Here's how the part is built. I have some questions about the finished solid (model axes, mm). A direction names the side the tool comes from. Coordinates: 2 decimals unless noted, no trailing zeros. Write each loop counter-clockwise with the first axis right and the second up, starting at its lowest first coordinate (ties: lowest second). Pieces come first, ordered by that corner, then holes.
from build123d import *

# Parameters (mm, degrees)
SKETCH2_W                = 100
SKETCH2_H                = 3
SKETCH2_H_2              = 11
BOSS_EXTRUDE2_DEPTH      = 2
SKETCH3_W                = 100
SKETCH3_H                = 3
BOSS_EXTRUDE3_DEPTH      = 20
FILLET2_R                = 1
BOSS_EXTRUDE5_DEPTH      = 30
BOSS_EXTRUDE5_DEPTH_BACK = 1
SKETCH5_W                = 9.5
SKETCH5_H                = 10
FILLET3_R                = 2
FILLET4_R                = 2
SKETCH6_R                = 2
CUT_EXTRUDE1_DEPTH       = 39
SKETCH7_R                = 2
CUT_EXTRUDE2_DEPTH       = 39


# Some blends are built 0.0001 mm under size
with BuildPart() as part:
    # Sketch2 → Boss-Extrude2 (new body)
    with BuildSketch(Plane(origin=(0, 0, 0), x_dir=(1, 0, 0), z_dir=(0, 1, 0))):
        with Locations((-50, 1.5)):
            Rectangle(SKETCH2_W, SKETCH2_H)
        with Locations((-50, -5.5)):
            Rectangle(SKETCH2_W, SKETCH2_H_2)
        with Locations((-50, -12.5)):
            Rectangle(SKETCH2_W, SKETCH2_H)
    extrude(amount=BOSS_EXTRUDE2_DEPTH)

    # Sketch3 → Boss-Extrude3 (add)
    with BuildSketch(Plane(origin=(0, 2, 0), x_dir=(1, 0, 0), z_dir=(0, 1, 0))):
        with Locations((-50, -12.5)):
            Rectangle(SKETCH3_W, SKETCH3_H)
        with Locations((-50, 1.5)):
            Rectangle(SKETCH3_W, SKETCH3_H)
    extrude(amount=BOSS_EXTRUDE3_DEPTH)

    # Fillet2
    fillet2_edges = [part.edges().sort_by_distance(p)[0] for p in [
        (-100, 11, -3),
        (0, 11, -3),
        (0, 11, 14),
        (-100, 11, 14),
        (-100, 2, 5.5),
        (0, 2, 5.5),
        (0, 12, 11),
        (-100, 12, 11),
        (-100, 22, 12.5),
        (0, 22, 12.5),
        (-50, 2, 11),
        (-50, 2, 0),
        (-100, 12, 0),
        (0, 12, 0),
        (-100, 22, -1.5),
        (0, 22, -1.5),
        (-50, 0, -3),
        (0, 0, 5.5),
        (-50, 0, 14),
        (-100, 0, 5.5),
    ]]
    fillet(fillet2_edges, radius=FILLET2_R - 0.0001)  # a hair under: the kernel refuses the full size

    # Sketch5 → Boss-Extrude5 (add, two sides: drawn at the far end of the back side and taken through both)
    with BuildSketch(Plane(origin=(0, 0, -3), x_dir=(-1, 0, 0), z_dir=(0, 0, -1)).offset(-BOSS_EXTRUDE5_DEPTH_BACK)):
        with Locations((50, 5)):
            Rectangle(SKETCH5_W, SKETCH5_H)
    extrude(amount=BOSS_EXTRUDE5_DEPTH + BOSS_EXTRUDE5_DEPTH_BACK)

    # Fillet3
    fillet3_edges = [part.edges().sort_by_distance(p)[0] for p in [
        (-45.25, 5, -33),
        (-50, 0, -33),
        (-54.75, 5, -33),
        (-50, 10, -33),
    ]]
    fillet(fillet3_edges, radius=FILLET3_R)

    # Fillet4
    # the kernel refuses this fillet: 2 mm, written as the material it adds along each edge
    with BuildSketch(Plane(origin=(-54.75, 0.9999, -2.0001), x_dir=(0, 0.0062831439655585564, -0.9999802608561371), z_dir=(0, -0.9999802608561371, -0.0062831439655585564))) as fillet4_piece_1_section:
        with BuildLine():
            CenterArc((-0.9999 - FILLET4_R, -FILLET4_R), FILLET4_R, 0, 90)
            Line((-0.9999, -FILLET4_R), (-0.9999, 0))
            Line((-0.9999, 0), (-0.9999 - FILLET4_R, 0))
        make_face()
    fillet4_piece_1 = revolve(axis=Axis((-54.75, 0.9999, -2.0001), (1, 0, 0)), revolution_arc=359.64, mode=Mode.PRIVATE)
    fillet4_piece_1 = split(fillet4_piece_1, bisect_by=Plane(origin=(-55.461006322, 0, -2.760267515), z_dir=(0, 1, 0)), keep=Keep.TOP, mode=Mode.PRIVATE)
    fillet4_piece_1 = split(fillet4_piece_1, bisect_by=Plane(origin=(-55.461006322, 0.239732481, 0), z_dir=(0, 0, -1)), keep=Keep.TOP, mode=Mode.PRIVATE)
    add(fillet4_piece_1)
    with BuildSketch(Plane(origin=(-45.25, 0.9999, -2.0001), x_dir=(0, 0.0062831439655585564, -0.9999802608561371), z_dir=(0, -0.9999802608561371, -0.0062831439655585564))) as fillet4_piece_2_section:
        with BuildLine():
            CenterArc((-0.9999 - FILLET4_R, FILLET4_R), FILLET4_R, 270, 90)
            Line((-0.9999, FILLET4_R), (-0.9999, 0))
            Line((-0.9999, 0), (-0.9999 - FILLET4_R, 0))
        make_face()
    fillet4_piece_2 = revolve(axis=Axis((-45.25, 0.9999, -2.0001), (1, 0, 0)), revolution_arc=359.64, mode=Mode.PRIVATE)
    fillet4_piece_2 = split(fillet4_piece_2, bisect_by=Plane(origin=(-44.538993678, 0, -2.760267519), z_dir=(0, 1, 0)), keep=Keep.TOP, mode=Mode.PRIVATE)
    fillet4_piece_2 = split(fillet4_piece_2, bisect_by=Plane(origin=(-44.538993678, 0.239732485, 0), z_dir=(0, 0, -1)), keep=Keep.TOP, mode=Mode.PRIVATE)
    add(fillet4_piece_2)
    with BuildSketch(Plane(origin=(-45.25, 10, -3), x_dir=(0, 0, -1), z_dir=(0, -1, 0)), Plane(origin=(-54.75, 0.9999, -3), x_dir=(0, 0, -1), z_dir=(0, 1, 0))) as fillet4_piece_3:
        with BuildLine():
            CenterArc((FILLET4_R, FILLET4_R), FILLET4_R, 180, 90)
            Line((0, FILLET4_R), (0, 0))
            Line((0, 0), (FILLET4_R, 0))
        make_face()
    extrude(amount=9.0001)

    # Sketch6 → Cut-Extrude1 (cut)
    with BuildSketch(Plane(origin=(0, 0, -3), x_dir=(-1, 0, 0), z_dir=(0, 0, -1))):
        with Locations((17.333333335, 18)):
            Circle(SKETCH6_R)
        with Locations((50.000000335, 18)):
            Circle(SKETCH6_R)
        with Locations((82.666667335, 18)):
            Circle(SKETCH6_R)
    extrude(amount=-CUT_EXTRUDE1_DEPTH, mode=Mode.SUBTRACT)

    # Sketch7 → Cut-Extrude2 (cut)
    with BuildSketch(Plane(origin=(0, 10, 0), x_dir=(1, 0, 0), z_dir=(0, 1, 0))):
        with Locations(Location((-50, 11, 0), (0, 0, 270))):
            Circle(SKETCH7_R)
    extrude(amount=-CUT_EXTRUDE2_DEPTH, mode=Mode.SUBTRACT)


solid = part.part
1. Thinking about a two-plate mould opening in Z: for faces 6 (the face through (-51, 11, 14)), 7 (the face through (-48.526, 19.352, 12.479)), 8 (the face through (-50, 5, -33)), 9 (the face through (-51, 12, 11)), which applies, pulls with the +Z half, pulls with the -Z half, needs draft (parallel to the pull), parting line crosses it, or undercut?
2. I want a section at D-D (x = -65). List the corners of the cut face in (y, z) for me.
3. For pin 1 Ø3 at (x, y) = (-50, 18) entering from -Z; pin 2 Ø3 at (y, z) = (3.5, -17.5) entering from -X; pin 3 Ø5 at (x, y) = (-42, 9.5) entering from -Z; pin 4 Ø4.5 at (x, y) = (-17.33, 18) entering from -Z, each with a flat end and sliding along its axis, tell me the tip position at first contact or that it passes through.
4. I want a section at B-B (z = -11). List the corners of the cut face in (x, y) for me.
5. I want a section at C-C (x = -50). List the corners of the cut face in (y, z) for me.
6. On a 3-axis mill with a long thin cutter (end or side, diameter ignored), from which of +Z, -Z, +X, -X, +Y, -Y can I reach the whole of each face in a straight line? I mean faces 1 (the face through (-54.75, 5, -18)), 2 (the face through (-45.25, 5, -18)), 3 (the face through (-51, 12, 0)), 4 (the face through (-19.24, 18.6, -1.52)), 5 (the face through (-50, 10, -17)). Say none if no direction works.
7. I want a section at A-A (y = 7). List the corners of the cut face in (x, z) for me.
8. If I drill on line 1 (Z direction, x = -43, y = 16.5); line 2 (Y direction, x = -50, z = 11.9); line 3 (Y direction, x = -51.5, z = -21.5), over which ranges is the centre line in solid material (lowest first)?
Response values:
1. face 6: pulls with the +Z half
1. face 7: needs draft
1. face 8: pulls with the -Z half
1. face 9: undercut
2. outline: (0, -2) arc R1 ccw to (1, -3) - (22, -3) - (22, 0) - (3, 0) arc R1 cw to (2, 1) - (2, 10) arc R1 cw to (3, 11) - (22, 11) - (22, 14) - (1, 14) arc R1 ccw to (0, 13) - close
3. pin 1: passes through
3. pin 2: stops at x = -54.75
3. pin 3: stops at z = -3.44
3. pin 4: stops at z = -3
4. outline: (-54.75, 0) - (-52, 0) - (-52, 10) - (-54.75, 10) - close; (-48, 0) - (-45.25, 0) - (-45.25, 10) - (-48, 10) - close
5. outline: (0, -31) arc R2 ccw to (2, -33) - (8, -33) arc R2 ccw to (10, -31) - (10, -13) - (0, -13) - close; (0, -9) - (10, -9) - (10, -3) - (16, -3) - (16, 0) - (3, 0) arc R1 cw to (2, 1) - (2, 10) arc R1 cw to (3, 11) - (16, 11) - (16, 14) - (1, 14) arc R1 ccw to (0, 13) - close; (20, -3) - (22, -3) - (22, 0) - (20, 0) - close; (20, 11) - (22, 11) - (22, 14) - (20, 14) - close
6. face 1: -Z, -X, +Y, -Y
6. face 2: -Z, +X, +Y, -Y
6. face 3: +X, -X, +Y
6. face 4: +Z, -Z
6. face 5: -Z, +X, -X, +Y
7. outline: (-100, -2) arc R1 ccw to (-99, -3) - (-56.75, -3) arc R2 cw to (-54.75, -5) - (-54.75, -31) arc R2 ccw to (-52.75, -33) - (-47.25, -33) arc R2 ccw to (-45.25, -31) - (-45.25, -5) arc R2 cw to (-43.25, -3) - (-1, -3) arc R1 ccw to (0, -2) - (0, -1) arc R1 ccw to (-1, 0) - (-99, 0) arc R1 ccw to (-100, -1) - close; (-100, 12) arc R1 ccw to (-99, 11) - (-1, 11) arc R1 ccw to (0, 12) - (0, 13) arc R1 ccw to (-1, 14) - (-99, 14) arc R1 ccw to (-100, 13) - close; hole circle Ø4 at (-50, -11)
8. line 1: z = -3 to 0, 11 to 14
8. line 2: y = 0 to 16, 20 to 22
8. line 3: y = 0 to 10
